```python
from build123d import *

# Parameters (mm, degrees)
IZIM1_R                     = 22.5
IZIM1_R_2                   = 10
Y_KSEKLIK_EKSTR_ZYON1_DEPTH = 30
Y_KSEKLIK_EKSTR_ZYON2_DEPTH = 5
Y_KSEKLIK_EKSTR_ZYON3_DEPTH = 20
IZIM4_W                     = 50
IZIM4_H                     = 20
KES_EKSTR_ZYON1_DEPTH       = 10
IZIM5_R                     = 4.5
KES_EKSTR_ZYON2_DEPTH       = 10


with BuildPart() as part:
    # Çizim1 → Yükseklik-Ekstrüzyon1 (new body)
    with BuildSketch(Plane(origin=(0, 0, 0), x_dir=(1, 0, 0), z_dir=(0, 1, 0))):
        with Locations(Location((0, 0, 0), (0, 0, 270))):
            Circle(IZIM1_R)
        with Locations(Location((0, 0, 0), (0, 0, 270))):
            Circle(IZIM1_R_2, mode=Mode.SUBTRACT)
    extrude(amount=Y_KSEKLIK_EKSTR_ZYON1_DEPTH)

    # Çizim2 → Yükseklik-Ekstrüzyon2 (add)
    with BuildSketch(Plane(origin=(0, 30, 0), x_dir=(1, 0, 0), z_dir=(0, 1, 0))):
        with BuildLine():
            Line((-6.614378278, 7.5), (-21.213203436, 7.5))
            ThreePointArc((-21.213203436, 7.5), (-22.5, 0), (-21.213203436, -7.5))
            Line((-21.213203436, -7.5), (-6.614378278, -7.5))
            ThreePointArc((-6.614378278, -7.5), (-10, 0), (-6.614378278, 7.5))
        make_face()
        with BuildLine():
            Line((21.213203436, 7.5), (6.614378278, 7.5))
            ThreePointArc((6.614378278, 7.5), (10, 0), (6.614378278, -7.5))
            Line((6.614378278, -7.5), (21.213203436, -7.5))
            ThreePointArc((21.213203436, -7.5), (22.5, 0), (21.213203436, 7.5))
        make_face()
    extrude(amount=Y_KSEKLIK_EKSTR_ZYON2_DEPTH)

    # Çizim3 → Yükseklik-Ekstrüzyon3 (add)
    with BuildSketch(Plane(origin=(0, 0, 0), x_dir=(1, 0, 0), z_dir=(0, 1, 0))):
        with BuildLine():
            Line((-14.142135624, -17.5), (-99.683227017, -17.5))
            Line((-99.683227017, -17.5), (-99.683227017, 17.5))
            Line((-99.683227017, 17.5), (-14.142135624, 17.5))
            ThreePointArc((-14.142135624, 17.5), (-18.371173071, 12.990381057), (-21.213203436, 7.5))
            ThreePointArc((-21.213203436, 7.5), (-22.5, 0), (-21.213203436, -7.5))
            ThreePointArc((-21.213203436, -7.5), (-18.371173071, -12.990381057), (-14.142135624, -17.5))
        make_face()
    extrude(amount=Y_KSEKLIK_EKSTR_ZYON3_DEPTH)

    # Çizim4 → Kes-Ekstrüzyon1 (cut)
    with BuildSketch(Plane(origin=(0, 20, 0), x_dir=(1, 0, 0), z_dir=(0, 1, 0))):
        with Locations((-74.683227017, 0)):
            Rectangle(IZIM4_W, IZIM4_H)
    extrude(amount=-KES_EKSTR_ZYON1_DEPTH, mode=Mode.SUBTRACT)

    # Çizim5 → Kes-Ekstrüzyon2 (cut)
    with BuildSketch(Plane(origin=(0, 10, 0), x_dir=(1, 0, 0), z_dir=(0, 1, 0))):
        with Locations(Location((-84.683227017, 0, 0), (0, 0, 270))):
            Circle(IZIM5_R)
        with Locations(Location((-64.683227017, 0, 0), (0, 0, 270))):
            Circle(IZIM5_R)
    extrude(amount=-KES_EKSTR_ZYON2_DEPTH, mode=Mode.SUBTRACT)


solid = part.part
```
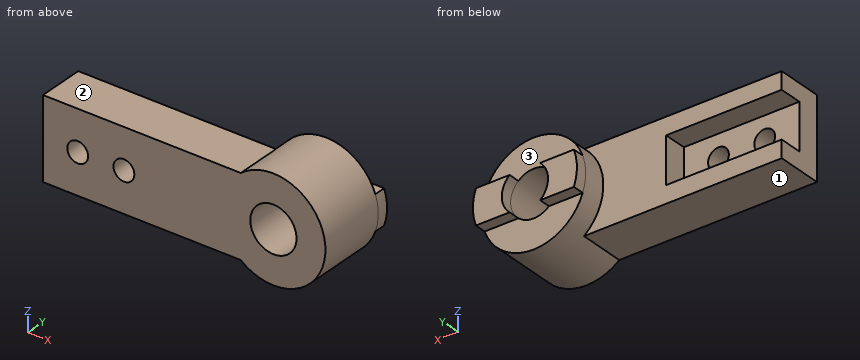
CAD build for the part. Positions are in the model's coordinates, mm. Face numbers are marked on the shaded views. A direction names the side the tool comes from. Coordinates: 2 decimals unless noted, no trailing zeros. Order: outer loops, then holes, each group sorted by start corner. A loop starts at its lowest first (then second) coordinate and runs counter-clockwise, first axis right, second up.
(1) Saw through at B-B, the plane x = 0. Write the cut outline in (y, z), and give its area (3 significant figures).
Solution:
outline: (0, -22.5) - (30, -22.5) - (30, -10) - (0, -10) - close; (0, 10) - (30, 10) - (30, 22.5) - (0, 22.5) - close
area: 750 mm2
(2) Saw through at D-D, the plane y = 14. Write the cut outline in (x, z), and give its area (3 significant figures).
Solution:
outline: (-99.68, -17.5) - (-14.14, -17.5) arc R22.5 ccw (long way) to (-14.14, 17.5) - (-99.68, 17.5) - (-99.68, 10) - (-49.68, 10) - (-49.68, -10) - (-99.68, -10) - close; hole circle Ø20 at (0, 0)
area: 3,070 mm2
(3) Saw through at A-A, the plane z = 0. Write the cut outline in (x, y).
Solution:
outline: (-99.68, 0) - (-89.18, 0) - (-89.18, 10) - (-99.68, 10) - close; (-80.18, 0) - (-69.18, 0) - (-69.18, 10) - (-80.18, 10) - close; (-60.18, 0) - (-10, 0) - (-10, 35) - (-22.5, 35) - (-22.5, 20) - (-49.68, 20) - (-49.68, 10) - (-60.18, 10) - close; (10, 0) - (22.5, 0) - (22.5, 35) - (10, 35) - close
(4) Which spindle directions (+Z, -Z, +X, -X, +Y, -Y) get a long thin tool onto all of the face, cutting with end or side? Do the marked faces 1, 2 and 3. Say none if no direction does.
Solution:
face 1: -Z, -X, +Y, -Y
face 2: +Z, -X, +Y, -Y
face 3: +Z, +X, -X, +Y
(5) Saw through at C-C, the plane y = 6.5. Write the cut outline in (x, z).
Solution:
outline: (-99.68, -17.5) - (-14.14, -17.5) arc R22.5 ccw (long way) to (-14.14, 17.5) - (-99.68, 17.5) - close; hole circle Ø9 at (-84.68, 0); hole circle Ø9 at (-64.68, 0); hole circle Ø20 at (0, 0)
(6) Pin check, flat tips, straight feed: pin 1 Ø5.5 at (x, z) = (-84.68, 0) entering from +Y; pin 2 Ø11 at (x, y) = (-66, 15.5) entering from -Z; pin 3 Ø1.5 at (y, z) = (21, -13) entering from -X; pin 4 Ø3 at (x, y) = (-72, 14.5) entering from +Z. Stop position of each tip, or through.
Solution:
pin 1: passes through
pin 2: stops at z = -17.5
pin 3: stops at x = -18.87
pin 4: stops at z = 17.5
(7) Drill centre lines: L1, parallel to X at y = 2, z = 0; L2, parallel to X at y = 23.75, z = 0; L3, parallel to X at y = 13.5, z = 0. Where is each one in solid material? Low to high.
Solution:
L1: x = -99.68 to -89.18, -80.18 to -69.18, -60.18 to -10, 10 to 22.5
L2: x = -22.5 to -10, 10 to 22.5
L3: x = -49.68 to -10, 10 to 22.5
